Source: three-view drawing plus pictorial views. Frame: mm from the lowest corner of the part. A direction names the side the tool comes from. Give positions to 0.01 mm unless a question says otherwise; leave off trailing zeros. Write each loop counter-clockwise with the first axis right and the second up, starting at its lowest first coordinate (ties: lowest second). Pieces come first, ordered by that corner, then holes.
Q1. Cut plane C-C on z = 16.5. Return the cut outline in (x, y), plus the area to 3 significant figures.
Q2. Cut plane A-A on y = 57.5. Return the cut outline in (x, z), plus the area to 3 significant figures.
Q3. Cut plane D-D on x = 23.5. Return the cut outline in (y, z), plus the area to 3 significant figures.
Q4. Cut plane B-B on x = 95. Return the cut outline in (y, z).
Q5. Line query: L1, parallel to X at y = 9, z = 114; L2, parallel to Y at x = 89, z = 17.5; L3, parallel to Z at x = 10, y = 59. Output: solid intervals per line, ascending.
Q6. Draft query along Z for the marked faces 1, 2, 3 and 4. Return one class per face: pulls with the +Z half, pulls with the -Z half, needs draft (parallel to the pull), parting line crosses it, or undercut.
Q7. Pin query (flat end, axial travel): pin 1 (10 mm diameter, centred on x = 142.5, y = 52.5, fed in from -Z); pin 2 (12 mm diameter, centred on x = 67, z = 77.5, fed in from -Y); pin 3 (5 mm diameter, centred on x = 160.5, z = 42, fed in from +Y) (3 decimals); pin 4 (6 mm diameter, centred on y = 46.5, z = 17.5, fed in from +X). Return the tip coordinate at first contact, or that it passes through.
Q8. Reachability of the marked faces 5, 6 and 7 from +Z, -Z, +X, -X, +Y, -Y: full face, straight path, thin tool, end or side. Return the list, or none.
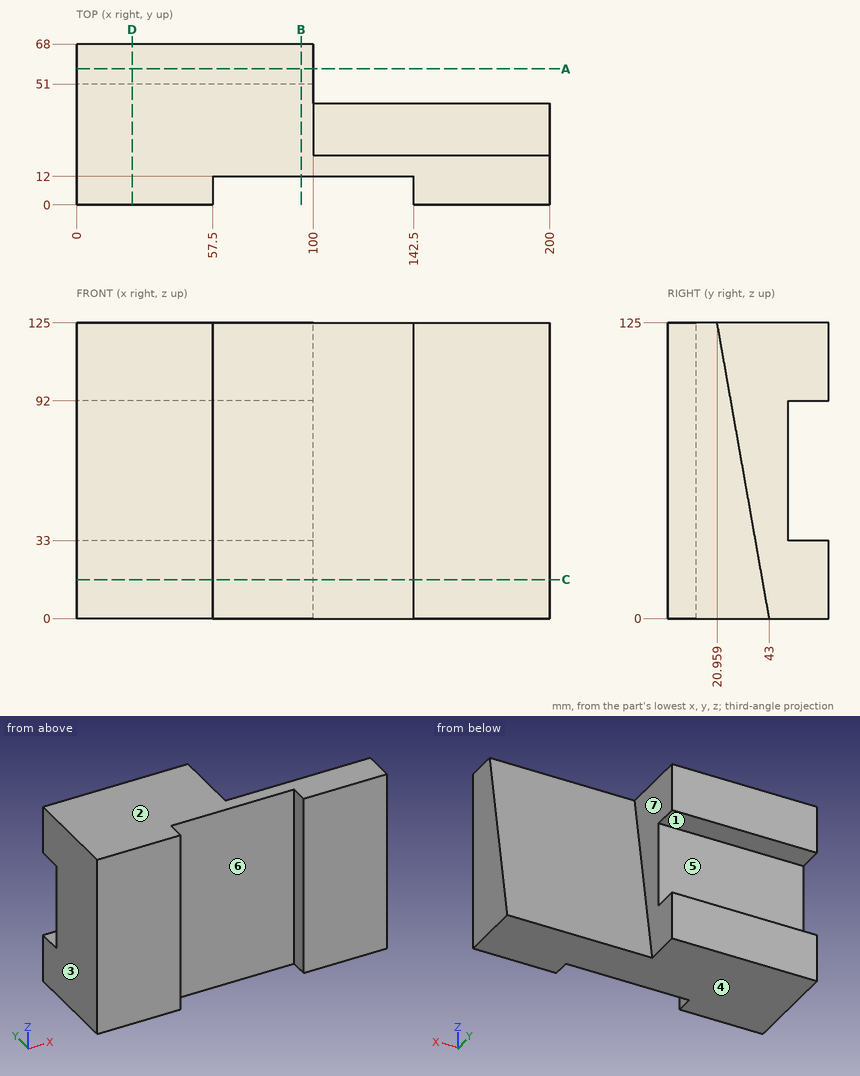
Data:
1. outline: (0, 0) - (57.5, 0) - (57.5, 12) - (142.5, 12) - (142.5, 0) - (200, 0) - (200, 40.09) - (100, 40.09) - (100, 68) - (0, 68) - close
1. area: 9,790 mm2
2. outline: (0, 0) - (100, 0) - (100, 33) - (0, 33) - close; (0, 92) - (100, 92) - (100, 125) - (0, 125) - close
2. area: 6,600 mm2
3. outline: (0, 0) - (68, 0) - (68, 33) - (51, 33) - (51, 92) - (68, 92) - (68, 125) - (0, 125) - close
3. area: 7,500 mm2
4. outline: (12, 0) - (68, 0) - (68, 33) - (51, 33) - (51, 92) - (68, 92) - (68, 125) - (12, 125) - close
5. L1: x = 0 to 57.5, 142.5 to 200
5. L2: y = 12 to 68
5. L3: z = 0 to 33, 92 to 125
6. face 1: undercut
6. face 2: pulls with the +Z half
6. face 3: needs draft
6. face 4: pulls with the -Z half
7. pin 1: passes through
7. pin 2: stops at y = 12
7. pin 3: stops at y = 36.035
7. pin 4: stops at x = 100
8. face 5: +X, -X, +Y
8. face 6: +Z, -Z, -Y
8. face 7: +Z, +X, +Y
